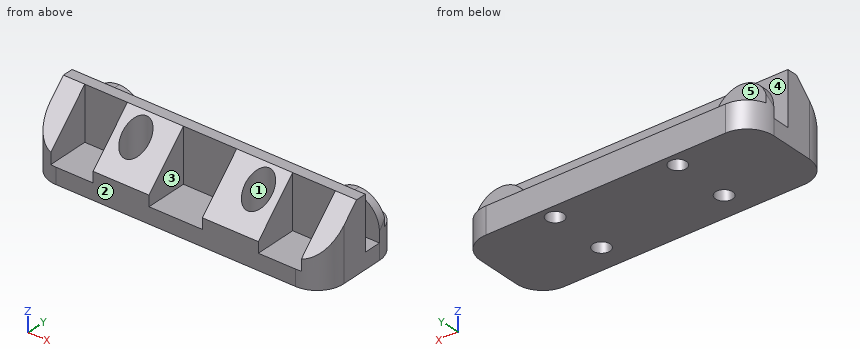
```python
from build123d import *

# Parameters (mm, degrees)
F0_W         = 55
F0_H         = 18.3
F1_DEPTH     = 3
F2_W         = 55
F2_H         = 5
F3_DEPTH     = 2
F4_W         = 55
F4_H         = 10
F5_DEPTH     = 1
F6_W         = 10
F6_H         = 1.5
F7_DEPTH     = 5
F8_R         = 4.99999
F9_DEPTH     = 9
F11_R        = 1.6
F12_DEPTH    = 5
F13_R        = 1.6
F14_DEPTH    = 13
F15_W        = 10
F15_H        = 8
F15_W_2      = 8
F16_DEPTH    = 10
F17_R        = 2.5
F18_DEPTH    = 9
F19_T1_DEPTH = 45.1469278075
F19_T3_DEPTH = 51.6469278075
F19_T5_DEPTH = 51.6469278075
F19_T7_DEPTH = 45.1469278075
F20_T1_DEPTH = 30


# Not quite as in the source:
# - a fillet or chamfer that OpenCascade refuses, or shapes differently, is made with other operations: its cross-section is extruded or revolved along the edge and cut away or added
# - a fillet or chamfer is up to 0.001 mm smaller than in the source, because OpenCascade refuses the exact size


with BuildPart() as f1:
    # F0 (on Top) → F1 (new body)
    with BuildSketch(Plane.XY):
        Rectangle(F0_W, F0_H)
    extrude(amount=F1_DEPTH)

    # F2 (on face) → F3 (join)
    with BuildSketch(Plane.XY.offset(3)):
        with Locations((0, 6.65)):
            Rectangle(F2_W, F2_H)
    extrude(amount=F3_DEPTH)

    # F4 (on face) → F5 (join)
    with BuildSketch(Plane.XY.offset(3)):
        with Locations((0, -4.15)):
            Rectangle(F4_W, F4_H)
    extrude(amount=F5_DEPTH)

    # F6 (on face) → F7 (join)
    with BuildSketch(Plane.XY.offset(5)):
        with Locations((22.5, 4.9)):
            Rectangle(F6_W, F6_H)
        with Locations((-22.5, 4.9)):
            Rectangle(F6_W, F6_H)
    extrude(amount=F7_DEPTH)

    # F8 (radius 5 in the source; OpenCascade refuses exactly that, so slightly less here)
    f8_edges = [f1.edges().sort_by_distance(p)[0] for p in [
        (17.5, 4.9, 10),
        (27.5, 4.9, 10),
        (-27.5, 4.9, 10),
        (-17.5, 4.9, 10),
    ]]
    fillet(f8_edges, radius=F8_R)

    # F9 (add): a face of the model
    f9_faces = [f1.faces().sort_by_distance(p)[0] for p in [
        (0, -4.15, 4),
    ]]
    extrude(f9_faces, amount=F9_DEPTH)

    # F11 (on face) → F12 (cut)
    with BuildSketch(Plane.XY.offset(5)):
        with Locations((11.5, 6.65)):
            Circle(F11_R)
        with Locations((-11.5, 6.65)):
            Circle(F11_R)
    extrude(amount=-F12_DEPTH, mode=Mode.SUBTRACT)

    # F13 (on face) → F14 (cut)
    with BuildSketch(Plane.XY.offset(13)):
        with Locations((11.5, -4.15)):
            Circle(F13_R)
        with Locations((-11.5, -4.15)):
            Circle(F13_R)
    extrude(amount=-F14_DEPTH, mode=Mode.SUBTRACT)

    # F15 (on face) → F16 (cut)
    with BuildSketch(Plane.XY.offset(13)):
        with Locations((0, -5.15)):
            Rectangle(F15_W, F15_H)
        with Locations((19.5, -5.15)):
            Rectangle(F15_W_2, F15_H)
        with Locations((-19.5, -5.15)):
            Rectangle(F15_W_2, F15_H)
    extrude(amount=-F16_DEPTH, mode=Mode.SUBTRACT)

    # F17 (on face) → F18 (cut)
    with BuildSketch(Plane.XY.offset(13)):
        with Locations((11.5, -4.15)):
            Circle(F17_R)
        with Locations((-11.5, -4.15)):
            Circle(F17_R)
    extrude(amount=-F18_DEPTH, mode=Mode.SUBTRACT)

    # F19: chamfer of 8 on 4 edges, made by hand

    # F19_s2 → F19_t1 (cut)
    with BuildSketch(Plane.YZ.offset(2.9265360963)):
        Polygon((-1.15, 13), (-9.15, 5), (-9.15, 13), align=None)
    extrude(amount=F19_T1_DEPTH, mode=Mode.SUBTRACT)

    # F19_s4 → F19_t3 (cut)
    with BuildSketch(Plane.YZ.offset(-15.5734639037)):
        Polygon((-1.15, 13), (-9.15, 5), (-9.15, 13), align=None)
    extrude(amount=F19_T3_DEPTH, mode=Mode.SUBTRACT)

    # F19_s6 → F19_t5 (cut)
    with BuildSketch(Plane.YZ.offset(-36.0734639037)):
        Polygon((-1.15, 13), (-9.15, 5), (-9.15, 13), align=None)
    extrude(amount=F19_T5_DEPTH, mode=Mode.SUBTRACT)

    # F19_s8 → F19_t7 (cut)
    with BuildSketch(Plane.YZ.offset(-48.0734639037)):
        Polygon((-1.15, 13), (-9.15, 5), (-9.15, 13), align=None)
    extrude(amount=F19_T7_DEPTH, mode=Mode.SUBTRACT)

    # F20: fillet of radius 5 on 4 edges, made by hand

    # F20_s2 → F20_t1 (cut)
    with BuildSketch(Plane.XY.offset(-12.5)):
        with BuildLine():
            ThreePointArc((22.5, -9.15), (26.0355339059, -7.6855339059), (27.5, -4.15))
            Line((27.5, -4.15), (27.5, -9.15))
            Line((27.5, -9.15), (22.5, -9.15))
        make_face()
        with BuildLine():
            ThreePointArc((22.5, 9.15), (26.0355339059, 7.6855339059), (27.5, 4.15))
            Line((27.5, 4.15), (27.5, 9.15))
            Line((27.5, 9.15), (22.5, 9.15))
        make_face()
        with BuildLine():
            ThreePointArc((-22.5, 9.15), (-26.0355339059, 7.6855339059), (-27.5, 4.15))
            Line((-27.5, 4.15), (-27.5, 9.15))
            Line((-27.5, 9.15), (-22.5, 9.15))
        make_face()
        with BuildLine():
            ThreePointArc((-22.5, -9.15), (-26.0355339059, -7.6855339059), (-27.5, -4.15))
            Line((-27.5, -4.15), (-27.5, -9.15))
            Line((-27.5, -9.15), (-22.5, -9.15))
        make_face()
    extrude(amount=F20_T1_DEPTH, mode=Mode.SUBTRACT)


solid = f1.part
```
The listing builds one solid part. Answer for the finished solid, in the listing's coordinates (mm). Face numbers are marked on the shaded views. A direction names the side the tool comes from. Round coordinates to 2 decimals unless told otherwise and drop trailing zeros. Write each loop counter-clockwise with the first axis right and the second up, starting at its lowest first coordinate (ties: lowest second). Pieces come first, ordered by that corner, then holes. Notation, with made-up numbers: (-1, 84.5) -> (10, 84.5) arc R13 cw to (10, 106.5) -> close; hole circle Ø9 at (14.25, -27). An arc over 180 degrees is marked (long way). Write item = value, one per line.
1) Given pin 1 (4 mm diameter, centred on y = -7, z = 6.5, fed in from +X); pin 2 (2 mm diameter, centred on x = -2.5, y = 7, fed in from +Z); pin 3 (1 mm diameter, centred on y = -5, z = 7, fed in from +X), each flat-ended and moving along its own axis, determine where each tip first touches the part or whether it passes through.
Check values:
pin_1 = 27.43
pin_2 = 5
pin_3 = 27.49
2) Section D-D on y = 6.65 is taken. Write down the section's boundary in (x, z), plus the area to 3 significant figures.
Check values:
outline = (-26.83, 0) -> (-13.1, 0) -> (-13.1, 5) -> (-26.83, 5) -> close; (-9.9, 0) -> (9.9, 0) -> (9.9, 5) -> (-9.9, 5) -> close; (13.1, 0) -> (26.83, 0) -> (26.83, 5) -> (13.1, 5) -> close
area = 236 mm²
3) Which of the six approach directions +Z, -Z, +X, -X, +Y, -Y give full straight-line access (tool end or side, diameter ignored) to the marked faces 1, 2, 3, 4 and 5?
Check values:
face_1 = +Z
face_2 = +Z, -Z, +X, -X, -Y
face_3 = +Z, -Y
face_4 = +Z, +X, -X
face_5 = +Z, +X, -X, +Y
4) Section A-A on x = -11.5 is taken. Write down the section's boundary in (y, z).
Check values:
outline = (-9.15, 0) -> (-5.75, 0) -> (-5.75, 4) -> (-6.65, 4) -> (-6.65, 7.5) -> (-9.15, 5) -> close; (-2.55, 0) -> (5.05, 0) -> (5.05, 5) -> (4.15, 5) -> (4.15, 3) -> (0.85, 3) -> (0.85, 13) -> (-1.15, 13) -> (-1.65, 12.5) -> (-1.65, 4) -> (-2.55, 4) -> close; (8.25, 0) -> (9.15, 0) -> (9.15, 5) -> (8.25, 5) -> close
5) Straight lines are drawn through the part: line 1 along X through (y, z) = (-4.15, 6.5); line 2 along Y through (x, z) = (-11.5, 1.55); line 3 along Y through (x, z) = (-18.5, 4.25). For each, find the intervals that lie inside material, in ascending order. Write a range as [from, to].
Check values:
line_1 = [-27.5, -23.5], [-15.5, -14], [-9, -5], [5, 9], [14, 15.5], [23.5, 27.5]
line_2 = [-9.15, -5.75], [-2.55, 5.05], [8.25, 9.15]
line_3 = [-1.15, 0.85], [4.15, 9.15]
6) Section B-B on z = 7 is taken. Write down the section's boundary in (x, y), plus the area to 3 significant figures.
Check values:
outline = (-27.5, -4.15) arc R5 ccw to (-26.5, -7.15) -> (-23.5, -7.15) -> (-23.5, -1.15) -> (-15.5, -1.15) -> (-15.5, -7.15) -> (-5, -7.15) -> (-5, -1.15) -> (5, -1.15) -> (5, -7.15) -> (15.5, -7.15) -> (15.5, -1.15) -> (23.5, -1.15) -> (23.5, -7.15) -> (26.5, -7.15) arc R5 ccw to (27.5, -4.15) -> (27.5, 0.85) -> (-27.5, 0.85) -> close; (-27.08, 4.15) -> (-17.92, 4.15) -> (-17.92, 5.65) -> (-27.08, 5.65) -> close; (17.92, 4.15) -> (27.08, 4.15) -> (27.08, 5.65) -> (17.92, 5.65) -> close; hole circle Ø5 at (-11.5, -4.15); hole circle Ø5 at (11.5, -4.15)
area = 270 mm²
7) Section C-C on x = 17 is taken. Write down the section's boundary in (y, z), plus the area to 3 significant figures.
Check values:
outline = (-9.15, 0) -> (9.15, 0) -> (9.15, 5) -> (4.15, 5) -> (4.15, 3) -> (0.85, 3) -> (0.85, 13) -> (-1.15, 13) -> (-1.15, 3) -> (-9.15, 3) -> close
area = 84.9 mm²
